```python
from build123d import *

# Parameters (mm, degrees)
F0_R     = 4.925
F1_DEPTH = 5.95
F2_R     = 3
F3_DEPTH = 95
F6_R     = 9.5
F7_DEPTH = 6


# Not quite as in the source:
# - a feature of the source that left no trace in its solid (it failed there, or was rolled back) is left out


with BuildPart() as f1:
    # F0 (on Top) → F1 (new body)
    with BuildSketch(Plane.XY):
        Circle(F0_R)
    extrude(amount=F1_DEPTH)

    # F2 (on face) → F3 (join)
    with BuildSketch(Plane.XY.offset(5.95)):
        Circle(F2_R)
    extrude(amount=F3_DEPTH)

    # F6 (on face) → F7 (join)
    with BuildSketch(Plane(origin=(-0.3810464275, 0, 19.0483774936), x_dir=(0.9997999772, 0, 0.0200001396), z_dir=(0.0200001396, 0, -0.9997999772))):
        with Locations((-0.7457245374, 0)):
            Circle(F6_R)
    extrude(amount=-F7_DEPTH)


solid = f1.part
```
Geometry check sheet. Reference: the model listing, model coordinates, mm. A direction names the side the tool comes from. Round coordinates to 2 decimals unless told otherwise and drop trailing zeros. Order: outer loops, then holes, each group sorted by start corner. A loop starts at its lowest first (then second) coordinate and runs counter-clockwise, first axis right, second up. Notation, with made-up numbers: (27.5, -6.75) - (55.5, -6.75) arc R20 ccw to (55.5, 6.25) - close; hole circle Ø5 at (-29, -31). An arc over 180 degrees is marked (long way). Use a Markdown table: item, result. Add a question column.
(1) Release check for a two-part mould opening along Z. For faces 1 (the flat face through (3.2, 0.1, 5.95)), 2 (the flat face through (0, 0, 0)), 3 (the cylindrical face through (-3, 0, 12)), 4 (the cylindrical face through (-3.908, -2.997, 2.933)) record: pulls with the +Z half, pulls with the -Z half, needs draft (parallel to the pull), parting line crosses it, or undercut.
(2) Material ranges on line 1 along Z through (x, y) = (3.5, -0.5); line 2 along Z through (x, y) = (-6, -4.25); line 3 along Y through (x, z) = (-2.75, 81), recorded low to high. Write a range as [from, to].
(3) Sectioned sample at B-B, the plane z = 11. Enter the section's corners in (x, y), and give its area (3 significant figures).
(4) Depth check by flat-ended pin: pin 1 (8 mm diameter, centred on y = -6, z = 33, fed in from -X); pin 2 (1.5 mm diameter, centred on x = 5, z = 39.5, fed in from -Y); pin 3 (3 mm diameter, centred on x = -8, y = 2.5, fed in from +Z); pin 4 (6 mm diameter, centred on x = -1, z = 84, fed in from +Y). Enter the tip coordinate at first touch or a pass-through.
(5) Sectioned sample at A-A, the plane y = 4. Enter the section's corners in (x, z).
(6) Sectioned sample at D-D, the plane y = 8.25. Enter the section's corners in (x, z).
(7) Sectioned sample at C-C, the plane y = 0. Enter the section's corners in (x, z) (3 decimals), and give its area (3 significant figures).
(8) Tool access check on faces 5 (the cylindrical face through (-3.245, 9.274, 21.95)), 6 (the flat face through (0, 0, 100.95)), 7 (the cylindrical face through (-3, 0, 62)). Record the directions out of +Z, -Z, +X, -X, +Y, -Y that give a thin tool (end or side, any length) a straight path to the whole face; none if there is none.
Answers below:
| question | item | result |
|---|---|---|
| 1 | face 1 | undercut |
| 1 | face 2 | pulls with the -Z half |
| 1 | face 3 | undercut |
| 1 | face 4 | needs draft |
| 2 | line 1 | [0, 5.95], [19.13, 25.13] |
| 2 | line 2 | [18.94, 24.94] |
| 2 | line 3 | [-1.2, 1.2] |
| 3 | outline | circle Ø6 at (0, 0) |
| 3 | area | 28.3 mm² |
| 4 | pin 1 | x = -2.24 |
| 4 | pin 2 | through |
| 4 | pin 3 | z = 24.93 |
| 4 | pin 4 | y = 3 |
| 5 | outline | (-9.86, 24.86) - (-9.74, 18.86) - (7.49, 19.21) - (7.37, 25.2) - close; (-2.87, 0) - (2.87, 0) - (2.87, 5.95) - (-2.87, 5.95) - close |
| 6 | outline | (-5.96, 24.94) - (-5.84, 18.94) - (3.58, 19.13) - (3.46, 25.13) - close |
| 7 | outline | (-10.745, 24.842) - (-10.625, 18.843) - (-3, 18.996) - (-3, 5.95) - (-4.925, 5.95) - (-4.925, 0) - (4.925, 0) - (4.925, 5.95) - (3, 5.95) - (3, 19.116) - (8.371, 19.223) - (8.251, 25.222) - (3, 25.117) - (3, 100.95) - (-3, 100.95) - (-3, 24.997) - close |
| 7 | area | 707 mm² |
| 8 | face 5 | none |
| 8 | face 6 | +Z, +X, -X, +Y, -Y |
| 8 | face 7 | +Z |
